from build123d import *

# Parameters (mm, degrees)
F1_DEPTH = 40
F2_R     = 3.5
F2_R_2   = 3.48483
F3_DEPTH = 25
F5_DEPTH = 25


with BuildPart() as f1:
    # F0 (on Front) → F1 (new body)
    with BuildSketch(Plane.XZ):
        Polygon((0, 0), (0, 40), (-9, 40), (-9, 0), (-9, -8), (17, -8), (17, 0), align=None)
    extrude(amount=F1_DEPTH)

    # F2 (on face) → F3 (cut)
    with BuildSketch(Plane.XY):
        with Locations((8.459888, -32.94181)):
            Circle(F2_R)
        with Locations((7.651556, -7.954882)):
            Circle(F2_R_2)
    extrude(amount=-F3_DEPTH, mode=Mode.SUBTRACT)

    # F4 (on face) → F5 (cut)
    with BuildSketch(Plane.YZ):
        with BuildLine():
            Line((-29.44, 10.001492), (-29.447151, 26.776387))
            ThreePointArc((-29.447151, 26.776387), (-32.855382, 30.498977), (-36.439575, 26.94549))
            Line((-36.439575, 26.94549), (-36.439575, 10.05451))
            Line((-36.439575, 10.05451), (-36.439575, 9.94549))
            ThreePointArc((-36.439575, 9.94549), (-32.911998, 6.500112), (-29.44, 10.001492))
        make_face()
        with BuildLine():
            Line((-36.439575, 9.94549), (-36.439575, 10.05451))
            ThreePointArc((-36.439575, 10.05451), (-36.44, 10), (-36.439575, 9.94549))
        make_face()
        with BuildLine():
            Line((-11.436366, 9.335628), (-11.436366, 10.664372))
            ThreePointArc((-11.436366, 10.664372), (-11.5, 10), (-11.436366, 9.335628))
        make_face()
        with BuildLine():
            Line((-11.436366, 26.335628), (-11.436366, 10.664372))
            Line((-11.436366, 10.664372), (-11.436366, 9.335628))
            ThreePointArc((-11.436366, 9.335628), (-7.659282, 6.516624), (-4.500028, 10.01409))
            Line((-4.500028, 10.01409), (-4.565691, 26.325079))
            Line((-4.565691, 26.325079), (-4.571236, 27.70255))
            ThreePointArc((-4.571236, 27.70255), (-8.019464, 30.499946), (-11.436366, 27.664372))
            Line((-11.436366, 27.664372), (-11.436366, 26.335628))
        make_face()
        with BuildLine():
            ThreePointArc((-11.436366, 27.664372), (-11.5, 27), (-11.436366, 26.335628))
            Line((-11.436366, 26.335628), (-11.436366, 27.664372))
        make_face()
        with BuildLine():
            Line((-4.571236, 27.70255), (-4.565691, 26.325079))
            ThreePointArc((-4.565691, 26.325079), (-4.500028, 27.01409), (-4.571236, 27.70255))
        make_face()
    extrude(amount=-F5_DEPTH, mode=Mode.SUBTRACT)


solid = f1.part
The listing builds one solid part. Answer for the finished solid, in the listing's coordinates (mm). A direction names the side the tool comes from. Coordinates: 2 decimals unless noted, no trailing zeros. Order: outer loops, then holes, each group sorted by start corner. A loop starts at its lowest first (then second) coordinate and runs counter-clockwise, first axis right, second up. Notation, with made-up numbers: (-26, 67.5) -> (18, 67.5) arc R18 ccw to (18, 73.5) -> close; hole circle Ø5 at (31.5, -28.5). An arc over 180 degrees is marked (long way). Answer in a Markdown table with one row per item. Add a question column.
Item 1: Find section C-C (x = 8.75). Write down the section's boundary in (y, z).
Item 2: Which of the six approach directions +Z, -Z, +X, -X, +Y, -Y give full straight-line access (tool end or side, diameter ignored) to faces 1 (the face through (-4, -11.436, 19)), 2 (the face through (4, -20, -8)), 3 (the face through (9, -20, 0))?
Item 3: Find section A-A (y = -9). Write down the section's boundary in (x, z), then the cut area to 3 significant figures.
Item 4: Find the intervals of material crossed by L1, parallel to Y at x = -6.25, z = 11.5; L2, parallel to X at y = -19, z = 35.5; L3, parallel to Z at x = 3.75, y = -10.5, in increasing order. Write a range as from..to.
Item 5: Find section D-D (y = -38). Write down the section's boundary in (x, z).
Item 6: Find section B-B (x = -2.25). Write down the section's boundary in (y, z), then the cut area to 3 significant figures.
Item 7: Determine the mould class of faces 4 (the face through (-4.44, -7.73, 6.51)), 5 (the face through (-4, -20, 40)), 6 (the face through (7.7, -36.36, -3.94)), 7 (the face through (-2, 0, 11)) for opening direction Y: +Y half, -Y half, draft (parallel to the pull), parting line (faces both ways), or undercut.
Item 8: Each of these flat-tipped pins is pushed along its axis until it touches: P1, Ø9, axis at x = 7.65, y = -7.95, coming from the +Z side; P2, Ø6.5, axis at x = 8.46, y = -32.94, coming from the -Z side; P3, Ø20, axis at y = -14.5, z = 15.5, coming from the +X side. Where does it stop, or does it pass through?
Result set:
| question | item | result |
|---|---|---|
| 1 | outline | (-40, -8) -> (-36.43, -8) -> (-36.43, 0) -> (-40, 0) -> close; (-29.45, -8) -> (-11.26, -8) -> (-11.26, 0) -> (-29.45, 0) -> close; (-4.65, -8) -> (0, -8) -> (0, 0) -> (-4.65, 0) -> close |
| 2 | face 1 | +X, -X |
| 2 | face 2 | -Z, +X, -X, +Y, -Y |
| 2 | face 3 | +Z, +X, +Y, -Y |
| 3 | outline | (-9, -8) -> (4.33, -8) -> (4.33, 0) -> (0, 0) -> (0, 6.65) -> (-9, 6.65) -> close; (-9, 30.35) -> (0, 30.35) -> (0, 40) -> (-9, 40) -> close; (10.98, -8) -> (17, -8) -> (17, 0) -> (10.98, 0) -> close |
| 3 | area | 301 mm² |
| 4 | L1 | y = -40..-36.44, -29.44..-11.44, -4.51..0 |
| 4 | L2 | x = -9..0 |
| 4 | L3 | z = -8..0 |
| 5 | outline | (-9, -8) -> (17, -8) -> (17, 0) -> (0, 0) -> (0, 40) -> (-9, 40) -> close |
| 6 | outline | (-40, -8) -> (0, -8) -> (0, 40) -> (-40, 40) -> close; hole (-36.44, 9.95) arc R3.5 ccw to (-29.44, 10) -> (-29.45, 26.78) arc R3.5 ccw (long way) to (-36.44, 26.95) -> (-36.44, 10.05) arc R3.5 ccw to start; hole (-11.44, 9.34) arc R3.5 ccw to (-4.5, 10.01) -> (-4.57, 26.33) arc R3.5 ccw to (-4.57, 27.7) arc R3.5 ccw to (-11.44, 27.66) arc R3.5 ccw to (-11.44, 26.34) -> (-11.44, 10.66) arc R3.5 ccw to start |
| 6 | area | 1,610 mm² |
| 7 | face 4 | undercut |
| 7 | face 5 | draft |
| 7 | face 6 | undercut |
| 7 | face 7 | +Y half |
| 8 | P1 | stops at z = 0 |
| 8 | P2 | passes through |
| 8 | P3 | stops at x = 0 |
